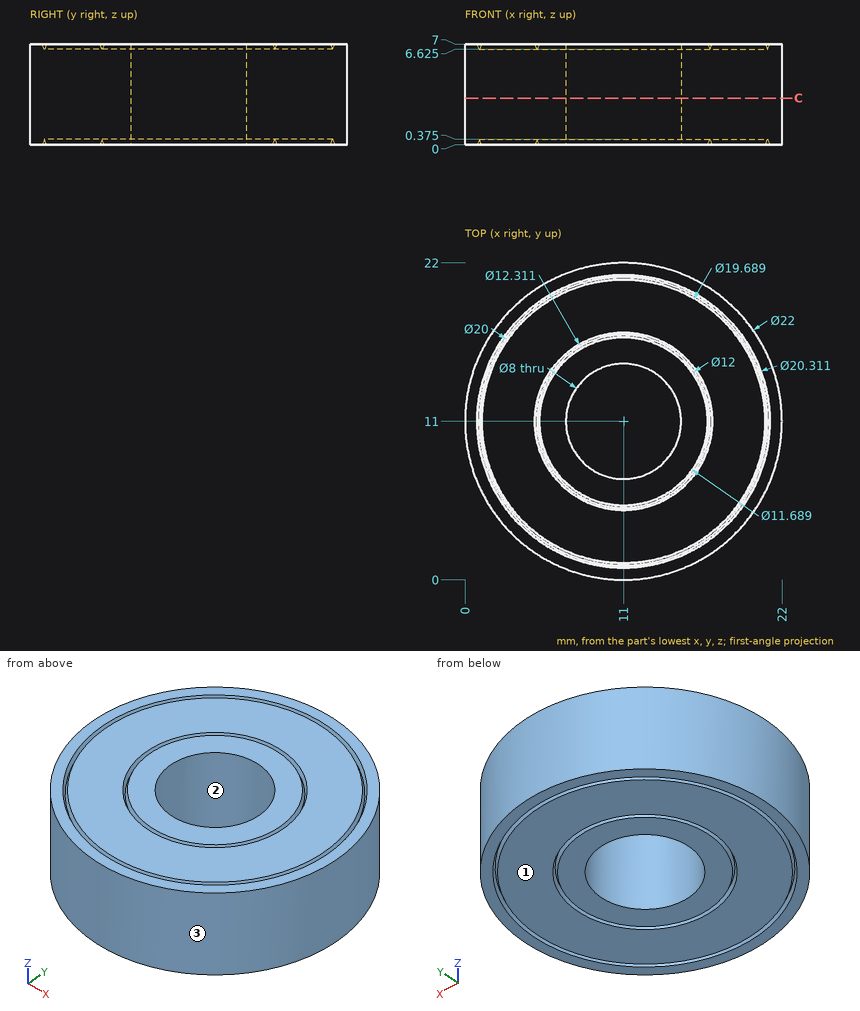
Answer from the drawing. Dimensions are ordinates in mm from the lowest x, y and z of the part. Round coordinates to 2 decimals unless told otherwise and drop trailing zeros. Write each loop counter-clockwise with the first axis right and the second up, starting at its lowest first coordinate (ties: lowest second). Pieces come first, ordered by that corner, then holes.
1. Straight lines are drawn through the part: L1, parallel to Y at x = 11, z = 4.25; L2, parallel to Y at x = 14.25, z = 6 (1 decimal); L3, parallel to X at y = 11.5, z = 4.5. For each, find the intervals that lie inside material, in ascending order.
2. Given pin 1 Ø1 at (x, z) = (8, 1) entering from -Y; pin 2 Ø1 at (x, z) = (4.5, 1.5) entering from -Y; pin 3 Ø3 at (y, z) = (16.5, 5.5) entering from -X, each flat-ended and moving along its own axis, determine where each tip first touches the part or whether it passes through.
3. Determine the mould class of the marked faces 1, 2 and 3 for opening direction X: pulls with the +X half, pulls with the -X half, needs draft (parallel to the pull), parting line crosses it, or undercut.
4. The part is cut by section C-C, the plane z = 3.25. Determine the outline of the cut face in (x, y).
Values:
1. L1: y = 0 to 7, 15 to 22
1. L2: y = 0.5 to 8.7, 13.3 to 21.5
1. L3: x = 0.01 to 7.03, 14.97 to 21.99
2. pin 1: stops at y = 0.29
2. pin 2: stops at y = 1.78
2. pin 3: stops at x = 0.75
3. face 1: needs draft
3. face 2: undercut
3. face 3: parting line crosses it
4. outline: circle Ø22 at (11, 11); hole circle Ø8 at (11, 11)
